Design review of the part built by this model. Coordinates are the model's own, in mm. Round coordinates to 2 decimals unless told otherwise and drop trailing zeros. Order: outer loops, then holes, each group sorted by start corner. A loop starts at its lowest first (then second) coordinate and runs counter-clockwise, first axis right, second up. Notation, with made-up numbers: (31.5, 58) - (54.5, 58) arc R6 cw to (54.5, 62) - close; hole circle Ø6 at (-25.75, 45). An arc over 180 degrees is marked (long way). Write item = value, one per line.
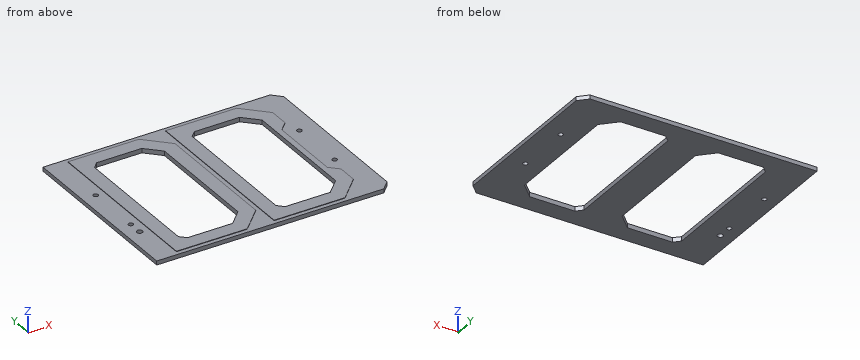
from build123d import *

# Parameters (mm, degrees)
SKETCH1_W           = 105.41
SKETCH1_H           = 82
SKETCH1_R           = 1.0795
SKETCH1_R_2         = 1.27
BOSS_EXTRUDE1_DEPTH = 1.778
BOSS_EXTRUDE2_DEPTH = 0.2
CUT_EXTRUDE1_DEPTH  = 2.978
CHAMFER1_SIZE       = 2.54
CHAMFER2_SIZE       = 3.81


with BuildPart() as part:
    # Sketch1 → Boss-Extrude1 (new body)
    with BuildSketch(Plane.XY):
        Rectangle(SKETCH1_W, SKETCH1_H)
        with Locations((44.45, 12.7)):
            Circle(SKETCH1_R, mode=Mode.SUBTRACT)
        with Locations((44.45, -12.7)):
            Circle(SKETCH1_R, mode=Mode.SUBTRACT)
        with Locations((-46.7106, 12.7)):
            Circle(SKETCH1_R, mode=Mode.SUBTRACT)
        with Locations((-46.7106, -12.7)):
            Circle(SKETCH1_R, mode=Mode.SUBTRACT)
        with Locations((-46.7106, -19.05)):
            Circle(SKETCH1_R_2, mode=Mode.SUBTRACT)
    extrude(amount=BOSS_EXTRUDE1_DEPTH)

    # Sketch2 → Boss-Extrude2 (add)
    with BuildSketch(Plane.XY.offset(1.778)):
        Polygon((-11, 39.095), (-1, 29.095), (-1, -29.095), (-11, -39.095), (-42.705, -39.095), (-42.705, 39.095), align=None)
        Polygon((42.705, 20.205), (38.895, 16.395), (38.895, -16.395), (42.705, -20.205), (42.705, -29.095), (32.705, -39.095), (1, -39.095), (1, 39.095), (32.705, 39.095), (42.705, 29.095), align=None)
    extrude(amount=BOSS_EXTRUDE2_DEPTH)

    # Sketch3 → Cut-Extrude1 (cut, through all)
    with BuildSketch(Plane.XY.offset(1.978)):
        Polygon((-36.355, -32.745), (-36.355, 32.745), (-13.630256121, 32.745), (-7.35, 26.464743879), (-7.35, -26.464743879), (-13.630256121, -32.745), align=None)
        Polygon((7.35, -32.745), (7.35, 32.745), (30.074743879, 32.745), (36.355, 26.464743879), (36.355, -26.464743879), (30.074743879, -32.745), align=None)
    extrude(amount=-CUT_EXTRUDE1_DEPTH, mode=Mode.SUBTRACT)

    # Chamfer1
    chamfer1_edges = [part.edges().sort_by_distance(p)[0] for p in [
        (-36.355, -32.745, 0.989),
        (-36.355, 32.745, 0.989),
        (7.35, -32.745, 0.989),
        (7.35, 32.745, 0.989),
    ]]
    chamfer(chamfer1_edges, length=CHAMFER1_SIZE)

    # Chamfer2
    chamfer2_edges = [part.edges().sort_by_distance(p)[0] for p in [
        (52.705, 41, 0.889),
        (52.705, -41, 0.889),
    ]]
    chamfer(chamfer2_edges, length=CHAMFER2_SIZE)


solid = part.part
1) We need section C-C on y = 12.7. Give the number of separate pieces and of enclosed holes in the cut face, and give its area (3 significant figures).
Findings:
separate_pieces = 5
enclosed_holes = 0
area = 80.9 mm^2
2) To check wall thickness, follow L1, parallel to Y at x = 44.45, z = 1.2; L2, parallel to X at y = -21.5, z = 0.8 (3 decimals); L3, parallel to Y at x = -26.5, z = 1.6 (3 decimals). State the ranges of each line that lie inside material, in increasing order. Write a range as from..to.
Findings:
L1 = -41..-13.78, -11.62..11.62, 13.78..41
L2 = -52.705..-36.355, -7.35..7.35, 36.355..52.705
L3 = -41..-32.745, 32.745..41
3) We need section D-D on y = -19.05. Write out the cut boundary in (x, z) (3 decimals), and give its area (3 significant figures).
Findings:
outline = (-52.705, 0) - (-47.981, 0) - (-47.981, 1.778) - (-52.705, 1.778) - close; (-45.441, 0) - (-36.355, 0) - (-36.355, 1.978) - (-42.705, 1.978) - (-42.705, 1.778) - (-45.441, 1.778) - close; (-7.35, 0) - (7.35, 0) - (7.35, 1.978) - (1, 1.978) - (1, 1.778) - (-1, 1.778) - (-1, 1.978) - (-7.35, 1.978) - close; (36.355, 0) - (52.705, 0) - (52.705, 1.778) - (41.55, 1.778) - (41.55, 1.978) - (36.355, 1.978) - close
area = 84.6 mm^2
4) Clearance check with flat-ended pins moving along their axes: pin 1 Ø1.9 at (x, y) = (-46.71, -12.7) entering from +Z; pin 2 Ø3 at (x, y) = (-46.71, 12.7) entering from +Z. State where each tip first meets the part, or that it passes through.
Findings:
pin_1 = through
pin_2 = 1.78
5) We need section A-A on y = 23. Write out the cut boundary in (x, z) (3 decimals), and give its area (3 significant figures).
Findings:
outline = (-52.705, 0) - (-36.355, 0) - (-36.355, 1.978) - (-42.705, 1.978) - (-42.705, 1.778) - (-52.705, 1.778) - close; (-7.35, 0) - (7.35, 0) - (7.35, 1.978) - (1, 1.978) - (1, 1.778) - (-1, 1.778) - (-1, 1.978) - (-7.35, 1.978) - close; (36.355, 0) - (52.705, 0) - (52.705, 1.778) - (42.705, 1.778) - (42.705, 1.978) - (36.355, 1.978) - close
area = 89.4 mm^2
6) We need section B-B on x = 44.45. Write out the cut boundary in (y, z), and give its area (3 significant figures).
Findings:
outline = (-41, 0) - (-13.78, 0) - (-13.78, 1.78) - (-41, 1.78) - close; (-11.62, 0) - (11.62, 0) - (11.62, 1.78) - (-11.62, 1.78) - close; (13.78, 0) - (41, 0) - (41, 1.78) - (13.78, 1.78) - close
area = 138 mm^2
